CAD build for the part. Positions are in the model's coordinates, mm. Coordinates: 2 decimals unless noted, no trailing zeros. Loops run counter-clockwise (first coordinate to the right, second up) from the corner with the lowest first, then second, coordinate; pieces in that order, holes last.
1) Wall check: line 1 along X through (y, z) = (-0.5, -68.25); line 2 along X through (y, z) = (-4.4, -63.5); line 3 along X through (y, z) = (-3.5, -62). Give the ranges that are in metal, low to high.
2) Saw through at A-A, the plane y = -3.2. Write the cut outline in (x, z).
3) Two-plate mould, pull along Z, no slides. Class faces 1 (the flat face through (4, -2, -60.668)), 2 (the cylindrical face through (75.916, -2.465, -66.796)), 3 (the flat face through (2, -5, -66)): +Z half, -Z half, draft (parallel to the pull), parting line (faces both ways), or undercut.
4) Pin check, flat tips, straight feed: pin 1 Ø1.5 at (y, z) = (-3, -63) entering from +X; pin 2 Ø1 at (y, z) = (-2, -69) entering from +X. Stop position of each tip, or through.
```python
from build123d import *

# Parameters (mm, degrees)
F0_R     = 2.893868
F0_R_2   = 2.944641
F1_DEPTH = 5
F2_R     = 6.542649
F3_DEPTH = 150


with BuildPart() as f1:
    # F0 (on Front) → F1 (new body)
    with BuildSketch(Plane.XZ):
        with BuildLine():
            ThreePointArc((-66.804364, -60.668005), (-71.804364, -65.668005), (-66.804364, -70.668005))
            Line((-66.804364, -70.668005), (73.195636, -70.668005))
            ThreePointArc((73.195636, -70.668005), (78.195636, -65.668005), (73.195636, -60.668005))
            Line((73.195636, -60.668005), (-66.804364, -60.668005))
        make_face()
        with Locations((-66.804364, -65.668005)):
            Circle(F0_R, mode=Mode.SUBTRACT)
        with Locations((73.195636, -65.668005)):
            Circle(F0_R_2, mode=Mode.SUBTRACT)
    extrude(amount=F1_DEPTH)


with BuildPart() as f3:
    # F2 (on Front) → F3 (new body)
    with BuildSketch(Plane.XZ):
        with Locations((-51.154699, 6.320113)):
            Circle(F2_R)
    extrude(amount=F3_DEPTH)


solid = f1.part
```
Data:
1. line 1: x = -71.09 to -68.11, -65.5 to 71.78, 74.61 to 77.48
1. line 2: x = -71.31 to -68.72, -64.89 to 71.2, 75.19 to 77.7
1. line 3: x = -70.2 to 76.59
2. outline: (-66.8, -70.67) - (73.2, -70.67) arc R5 ccw to (73.2, -60.67) - (-66.8, -60.67) arc R5 ccw to start; hole circle Ø5.79 at (-66.8, -65.67); hole circle Ø5.89 at (73.2, -65.67)
3. face 1: +Z half
3. face 2: undercut
3. face 3: draft
4. pin 1: stops at x = 77.81
4. pin 2: stops at x = 77.32
